```python
from build123d import *

# Parameters (mm, degrees)
F1_DEPTH = 3
F2_W     = 15
F2_H     = 3
F3_DEPTH = 3


with BuildPart() as f1:
    # F0 (on Top) → F1 (new body)
    with BuildSketch(Plane.XY):
        with BuildLine():
            Line((20, 30), (-20, 30))
            ThreePointArc((-20, 30), (-41.213203, 21.213203), (-50, 0))
            ThreePointArc((-50, 0), (-41.213203, -21.213203), (-20, -30))
            Line((-20, -30), (20, -30))
            ThreePointArc((20, -30), (41.213203, -21.213203), (50, 0))
            ThreePointArc((50, 0), (41.213203, 21.213203), (20, 30))
        make_face()
    extrude(amount=F1_DEPTH)

    # F2 (on face) → F3 (join)
    with BuildSketch(Plane.XY.offset(3)):
        with Locations((0, 28.5)):
            Rectangle(F2_W, F2_H)
        with BuildLine():
            Line((-47, 7.5), (-49.047375, 7.5))
            ThreePointArc((-49.047375, 7.5), (-49.760891, 3.780129), (-50, 0))
            ThreePointArc((-50, 0), (-49.760891, -3.780129), (-49.047375, -7.5))
            Line((-49.047375, -7.5), (-47, -7.5))
            Line((-47, -7.5), (-47, 7.5))
        make_face()
        with Locations((0, -28.5)):
            Rectangle(F2_W, F2_H)
        with BuildLine():
            ThreePointArc((50, 0), (49.760891, 3.780129), (49.047375, 7.5))
            Line((49.047375, 7.5), (47, 7.5))
            Line((47, 7.5), (47, -7.5))
            Line((47, -7.5), (49.047375, -7.5))
            ThreePointArc((49.047375, -7.5), (49.760891, -3.780129), (50, 0))
        make_face()
    extrude(amount=F3_DEPTH)


solid = f1.part
```
Source: CAD feature listing. Evaluate the final solid. Frame: model axes, mm. A direction names the side the tool comes from. Coordinates: 2 decimals unless noted, no trailing zeros. Write each loop counter-clockwise with the first axis right and the second up, starting at its lowest first coordinate (ties: lowest second). Pieces come first, ordered by that corner, then holes. Notation, with made-up numbers: M 12,12 L 65,12 A24 cw 65,29 Z; hole C 74,18 d4. An arc over 180 degrees is marked long. Answer as a JSON object with one key per item and string values.
1. Cut plane C-C on y = -6.5. Output: boundary loops of the cut face in (x, z), plus the area to 3 significant figures.
Evaluation:
{"outline": "M -49.29,0 L 49.29,0 L 49.29,6 L 47,6 L 47,3 L -47,3 L -47,6 L -49.29,6 Z", "area": "309 mm^2"}
2. Ray query, L1, parallel to Y at x = -2.5, z = 4.15; L2, parallel to Z at x = -32.5, y = 1; L3, parallel to Y at x = -40, z = 1.5. Return the intervals inside material, ascending.
Evaluation:
{"L1": "-30 to -27, 27 to 30", "L2": "0 to 3", "L3": "-22.36 to 22.36"}
3. Cut plane A-A on z = 1.9. Output: boundary loops of the cut face in (x, y).
Evaluation:
{"outline": "M -50,0 A30 ccw -20,-30 L 20,-30 A30 ccw 50,0 A30 ccw 20,30 L -20,30 A30 ccw Z"}
4. Draft query along X for faces 5 (the flat face through (47, 0, 4)), 6 (the flat face through (0, 29, 6)), 7 (the flat face through (7.5, -29, 4)). Return one class per face: released by +X, released by -X, zero draft, split by the parting line, or undercut.
Evaluation:
{"face 5": "undercut", "face 6": "zero draft", "face 7": "released by +X"}
5. Access query for faces 1 (the flat face through (48, 7.5, 4)), 2 (the flat face through (-47, 0, 4)), 3 (the flat face through (48, -7.5, 4)), 4 (the flat face through (-7.5, -29, 4)). Directions: +Z, -Z, +X, -X, +Y, -Y. A direction counts if a zero-diameter tool reaches every point of the face in a straight line with its end or side. Return the directions, or none.
Evaluation:
{"face 1": "+Z, +X, -X, +Y", "face 2": "+Z, +Y, -Y", "face 3": "+Z, +X, -X, -Y", "face 4": "+Z, -X, +Y, -Y"}
6. Contact query for flat-ended pins moving along their axis: P1, Ø0.6, axis at x = 48.5, z = 5, coming from the +Y side; P2, Ø3.5, axis at y = 2.5, z = 5, coming from the -X side; P3, Ø3.5, axis at y = 3, z = 4.5, coming from the +X side; P4, Ø8, axis at x = 7, y = 23.5, coming from the -Z side. Output: stop coordinate, or through.
Evaluation:
{"P1": "y = 7.5", "P2": "x = -49.99", "P3": "x = 49.97", "P4": "z = 0"}
7. Cut plane B-B on x = 0.5. Output: boundary loops of the cut face in (y, z).
Evaluation:
{"outline": "M -30,0 L 30,0 L 30,6 L 27,6 L 27,3 L -27,3 L -27,6 L -30,6 Z"}
8. Cut plane D-D on x = -12. Output: boundary loops of the cut face in (y, z).
Evaluation:
{"outline": "M -30,0 L 30,0 L 30,3 L -30,3 Z"}
